Geometry check sheet. Reference: the model listing, model coordinates, mm. A direction names the side the tool comes from. Give positions to 0.01 mm unless a question says otherwise; leave off trailing zeros. Loops run counter-clockwise (first coordinate to the right, second up) from the corner with the lowest first, then second, coordinate; pieces in that order, holes last. Notation, with made-up numbers: (-31, 44.5) - (-17, 44.5) arc R23 ccw to (-17, 75.5) - close; hole circle Ø3 at (37.25, 66). An arc over 180 degrees is marked (long way). Use a Markdown table: item, result. Add a question column.
1. Set-up check for faces 4 (the flat face through (-7, 0, 21.05)), 5 (the cylindrical face through (-7.607, -0.021, 25.094)), 6 (the flat face through (5.527, 0.021, 8.946)): record each of +Z, -Z, +X, -X, +Y, -Y from which the full face is reachable in a straight line by a thin tool's end or side.
2. Cross-section at D-D on z = 1.5. Enter the section's corners in (x, y).
3. Draft check along X on faces 1 (the flat face through (-5.608, 0, 25)), 2 (the flat face through (-5.63, -0.02, 20.07)), 3 (the flat face through (19.58, -0.02, 24.47)). Enter one of: pulls with the +X half, pulls with the -X half, needs draft (parallel to the pull), parting line crosses it, or undercut.
4. Cross-section at B-B on x = 0. Enter the section's corners in (y, z).
5. Material ranges on L1, parallel to X at y = 0.2, z = -3.45; L2, parallel to X at y = 0.1, z = -5; L3, parallel to Z at x = -1.75, y = -1, recorded low to high.
6. Depth check by flat-ended pin: P1, Ø1, axis at y = 0.5, z = 16.5, coming from the -X side; P2, Ø4, axis at x = 13.5, z = 20.5, coming from the +Y side; P3, Ø1, axis at y = 1, z = 8, coming from the +X side; P4, Ø1.5, axis at x = 15.5, y = -0.5, coming from the -Z side. Enter the tip coordinate at first touch or a pass-through.
7. Cross-section at C-C on y = 0.1. Count the separate pieces of the cut face and the enclosed holes in it, and give its area (3 significant figures).
8. Cross-section at A-A on z = -3.45. Enter the section's corners in (x, y).
from build123d import *
from OCP.BRepFilletAPI import BRepFilletAPI_MakeChamfer, BRepFilletAPI_MakeFillet

# Parameters (mm, degrees)
SKETCH1_R               = 3.45
BOSS_EXTRUDE1_DEPTH     = 1.5
BOSS_EXTRUDE2_DEPTH     = 1.5
CUT_EXTRUDE1_DEPTH      = 36.300885258
CUT_EXTRUDE1_DEPTH_BACK = 36.300885258
SKETCH3_W               = 12
SKETCH3_H               = 3
CHAMFER5_SIZE           = 2
FILLET6_R               = 4
FILLET6_R_2             = 1.5
CHAMFER6_SIZE           = 2
CUT_EXTRUDE2_DEPTH      = 36.300885258
CUT_EXTRUDE2_DEPTH_BACK = 36.300885258
CHAMFER7_SIZE           = 2
CHAMFER7_SIZE2          = 1.864165933


with BuildPart() as part:
    # Sketch1 → Boss-Extrude1 (new, symmetric)
    with BuildSketch(Plane(origin=(0, 0, 0), x_dir=(1, 0, 0), z_dir=(0, 1, 0))):
        with BuildLine():
            Line((-4, -29.05), (-6.431473945, 2.961489101))
            ThreePointArc((-6.431473945, 2.961489101), (0, 9.9), (6.431473945, 2.961489101))
            Line((6.431473945, 2.961489101), (4, -29.05))
            Line((4, -29.05), (-4, -29.05))
        make_face()
        with Locations(Location((0, 3.45, 0), (0, 0, 270))):
            Circle(SKETCH1_R, mode=Mode.SUBTRACT)
    extrude(amount=BOSS_EXTRUDE1_DEPTH, both=True)

    # Sketch2 → Boss-Extrude2 (add, symmetric)
    with BuildSketch(Plane(origin=(0, 0, 0), x_dir=(1, 0, 0), z_dir=(0, 1, 0))):
        Polygon((-4.607650319, -21.05), (-4, -29.05), (-9.607650319, -29.05), (-9.607650319, -21.05), align=None)
        Polygon((4.455737739, -23.05), (20, -23.05), (20, -29.05), (4, -29.05), align=None)
    extrude(amount=BOSS_EXTRUDE2_DEPTH, both=True)

    # Sketch3 → Cut-Extrude1 (cut, two sides: drawn at the far end of the back side and taken through both)
    with BuildSketch(Plane(origin=(0, 0, 0), x_dir=(1, 0, 0), z_dir=(0, 1, 0)).offset(-CUT_EXTRUDE1_DEPTH_BACK)):
        with Locations((14, -27.55)):
            Rectangle(SKETCH3_W, SKETCH3_H)
    extrude(amount=CUT_EXTRUDE1_DEPTH + CUT_EXTRUDE1_DEPTH_BACK, mode=Mode.SUBTRACT)

    # Chamfer5
    chamfer5_edges = [part.edges().sort_by_distance(p)[0] for p in [
        (20, 0, 26.05),
    ]]
    chamfer(chamfer5_edges, length=CHAMFER5_SIZE)

    # Fillet6
    fillet6_edges_1 = [part.edges().sort_by_distance(p)[0] for p in [
        (18, 0, 26.05),
    ]]
    fillet6_edges_2 = [part.edges().sort_by_distance(p)[0] for p in [
        (8, 0, 26.05),
        (8, 0, 29.05),
    ]]
    fillet6 = BRepFilletAPI_MakeFillet(part.part.solid().wrapped)
    for e in fillet6_edges_1:
        fillet6.Add(FILLET6_R - 0.0001, e.wrapped)
    for e in fillet6_edges_2:
        fillet6.Add(FILLET6_R_2 - 0.0001, e.wrapped)
    add(Compound.cast(fillet6.Shape()), mode=Mode.REPLACE)  # a hair under: the kernel refuses the full size

    # Chamfer6
    chamfer6_edges = [part.edges().sort_by_distance(p)[0] for p in [
        (-9.607650319, 0, 21.05),
        (-9.607650319, 0, 29.05),
    ]]
    chamfer(chamfer6_edges, length=CHAMFER6_SIZE)

    # Sketch4 → Cut-Extrude2 (cut, two sides: drawn at the far end of the back side and taken through both)
    with BuildSketch(Plane(origin=(0, 0, 0), x_dir=(1, 0, 0), z_dir=(0, 1, 0)).offset(-CUT_EXTRUDE2_DEPTH_BACK)):
        with BuildLine():
            Line((-5.607650319, -23.05), (-5.607650319, -27.05))
            ThreePointArc((-5.607650319, -27.05), (-7.607650319, -25.05), (-5.607650319, -23.05))
        make_face()
    extrude(amount=CUT_EXTRUDE2_DEPTH + CUT_EXTRUDE2_DEPTH_BACK, mode=Mode.SUBTRACT)

    # Chamfer7: one chamfer whose edges measure the first distance from different faces: ONE call of the kernel's chamfer builder (chamfer() names one face for all edges)
    chamfer7_edges_1 = [part.edges().sort_by_distance(p)[0] for p in [
        (4.455737739, 0, 23.05),
    ]]
    chamfer7_side_1 = [part.faces().sort_by_distance(p)[0] for p in [
        (12.22786887, 0, 23.05),
    ]]
    chamfer7_edges_2 = [part.edges().sort_by_distance(p)[0] for p in [
        (-4.607650319, 0, 21.05),
    ]]
    chamfer7_side_2 = [part.faces().sort_by_distance(p)[0] for p in [
        (-5.519562132, 0, 9.04425545),
    ]]
    chamfer7 = BRepFilletAPI_MakeChamfer(part.part.solid().wrapped)
    for e in chamfer7_edges_1:
        chamfer7.Add(CHAMFER7_SIZE, CHAMFER7_SIZE2, e.wrapped, chamfer7_side_1[0].wrapped)  # the first distance lies on this face
    for e in chamfer7_edges_2:
        chamfer7.Add(CHAMFER7_SIZE, CHAMFER7_SIZE2, e.wrapped, chamfer7_side_2[0].wrapped)  # the first distance lies on this face
    add(Compound.cast(chamfer7.Shape()), mode=Mode.REPLACE)


solid = part.part
Values found:
| question | item | result |
|---|---|---|
| 1 | face 4 | -Z, -X, +Y, -Y |
| 1 | face 5 | +Y, -Y |
| 1 | face 6 | +X, +Y, -Y |
| 2 | outline | (-6.09, -1.5) - (6.09, -1.5) - (6.09, 1.5) - (-6.09, 1.5) - close |
| 3 | face 1 | undercut |
| 3 | face 2 | pulls with the -X half |
| 3 | face 3 | pulls with the +X half |
| 4 | outline | (-1.5, -9.9) - (1.5, -9.9) - (1.5, -6.9) - (-1.5, -6.9) - close; (-1.5, 0) - (1.5, 0) - (1.5, 29.05) - (-1.5, 29.05) - close |
| 5 | L1 | x = -6.45 to -3.45, 3.45 to 6.45 |
| 5 | L2 | x = -6.26 to -3.08, 3.08 to 6.26 |
| 5 | L3 | z = -9.66 to -6.42, -0.48 to 29.05 |
| 6 | P1 | stops at x = -4.99 |
| 6 | P2 | passes through |
| 6 | P3 | stops at x = 5.64 |
| 6 | P4 | stops at z = 23.05 |
| 7 | separate pieces | 1 |
| 7 | enclosed holes | 2 |
| 7 | area | 460 mm2 |
| 8 | outline | (-6.45, -1.5) - (-3.45, -1.5) - (-3.45, 1.5) - (-6.45, 1.5) - close; (3.45, -1.5) - (6.45, -1.5) - (6.45, 1.5) - (3.45, 1.5) - close |
